Could you check a few things on this drawing? It's one solid part, dimensions in mm from its lowest x, y, z. Give positions to 0.01 mm unless a question says otherwise; leave off trailing zeros. Write item = value, one per line.
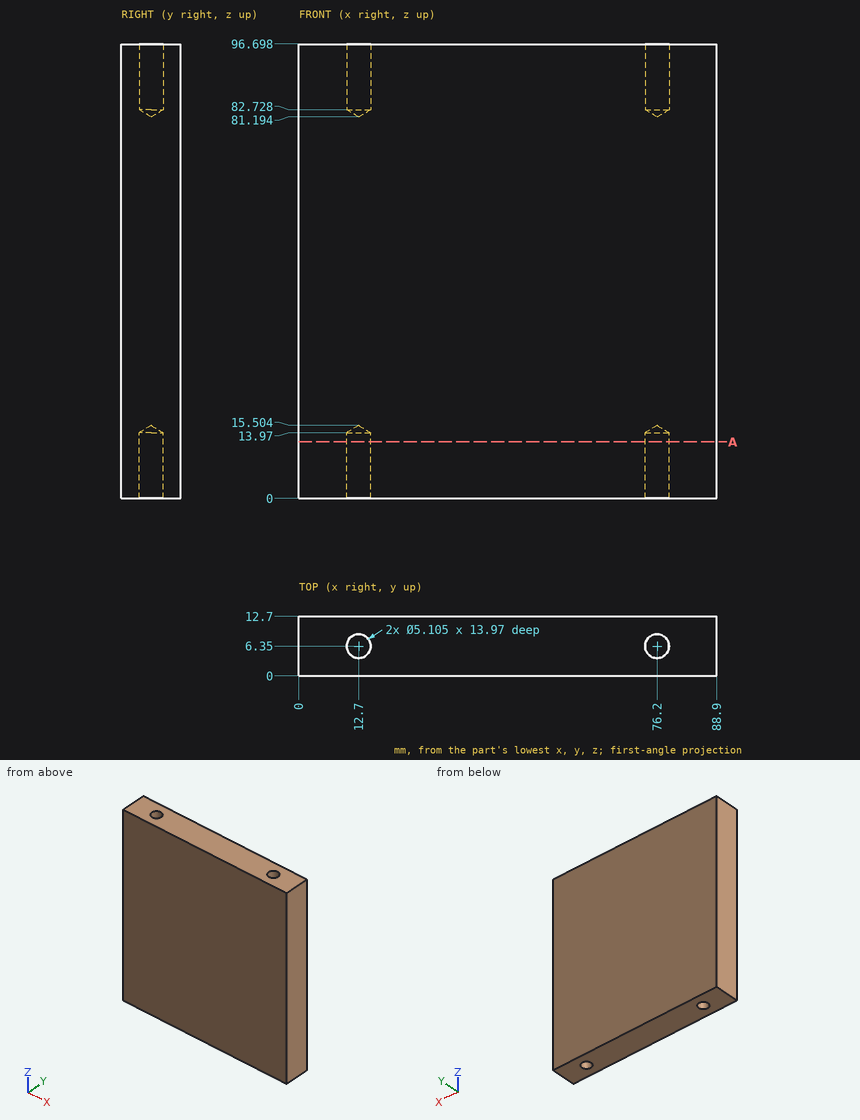
Q1. I need wall thicknesses on L1, parallel to X at y = 6.35, z = 93.5; L2, parallel to Y at x = 76.2, z = 92; L3, parallel to Z at x = 15, y = 7. Which ranges of each line are inside material? Lowest first, please.
Output:
L1 = 0 to 10.15, 15.25 to 73.65, 78.75 to 88.9
L2 = 0 to 3.8, 8.9 to 12.7
L3 = 14.07 to 82.63
Q2. For pin 1 (4 mm diameter, centred on x = 33.5, y = 3, fed in from -Z); pin 2 (3 mm diameter, centred on x = 12.7, y = 6.35, fed in from -Z), each with a flat end and sliding along its axis, tell me the tip position at first contact or that it passes through.
Output:
pin_1 = 0
pin_2 = 14.6
Q3. Imagine slicing it at A-A, the plane z = 12. Give the number of separate pieces and of enclosed holes in the cut face, then the cut area to 3 significant figures.
Output:
separate_pieces = 1
enclosed_holes = 2
area = 1,090 mm2
